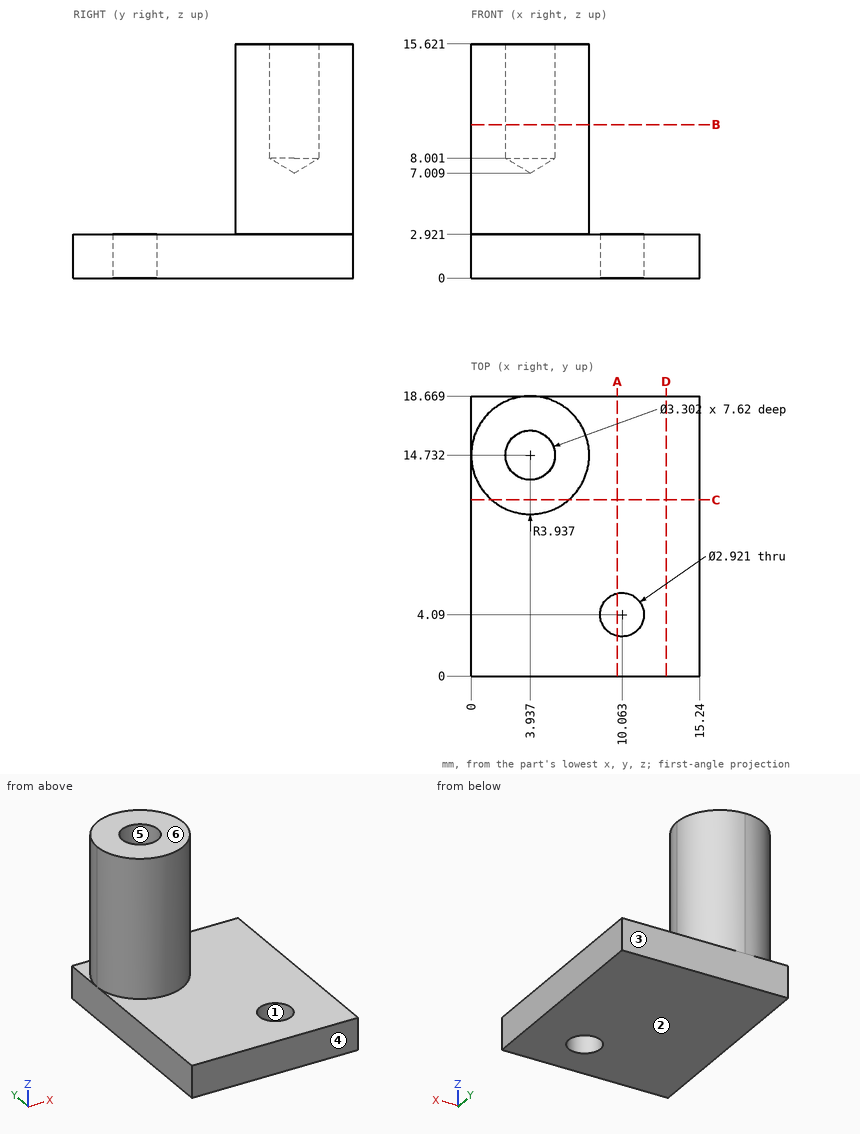
Job drawing, mm, ordinate dimensions from the low corner. One solid piece. A direction names the side the tool comes from. Round coordinates to 2 decimals unless told otherwise and drop trailing zeros. Loops run counter-clockwise (first coordinate to the right, second up) from the corner with the lowest first, then second, coordinate; pieces in that order, holes last. Notation, with made-up numbers: (87, -9) -> (119, -9) arc R25 cw to (119, 12) -> close; hole circle Ø6 at (-39, -25.5). An arc over 180 degrees is marked (long way). One line per item, written item: value. Start each with the question number.
Q1. Probe line 1 along Z through (x, y) = (12, 10.5); line 2 along X through (y, z) = (15.5, 7.75) (1 decimal); line 3 along X through (y, z) = (15, 8.75) (1 decimal). List the from-to ranges inside material, lowest first.
Q2. Two-plate mould, pull along Y, no slides. Class the marked faces 1, 2, 3 and 4: released by +Y, released by -Y, zero draft, split by the parting line, or undercut.
Q3. Cut at D-D on x = 13. List the corners of the cut face in (y, z).
Q4. Cut at B-B on z = 10.25. List the corners of the cut face in (x, y).
Q5. Cut at C-C on y = 11.75. List the corners of the cut face in (x, z).
Q6. 3-axis set-ups, long thin cutter, end or side, ignore diameter. For the marked faces 5 and 6: which of +Z, -Z, +X, -X, +Y, -Y reach the whole face in a straight line?
Q7. Cut at A-A on x = 9.75. List the corners of the cut face in (y, z).
Q8. Drop flat-ended pins along their axis: pin 1 Ø2 at (x, z) = (3, 6.5) entering from +Y; pin 2 Ø6 at (x, y) = (12.5, 12.5) entering from +Z; pin 3 Ø1.5 at (y, z) = (11, 11) entering from -X. Give the stop position or say it passes through.
Computed:
1. line 1: 0 to 2.92
1. line 2: 0.1 to 3, 4.9 to 7.8
1. line 3: 0 to 2.3, 5.6 to 7.9
2. face 1: undercut
2. face 2: zero draft
2. face 3: released by +Y
2. face 4: released by -Y
3. outline: (0, 0) -> (18.67, 0) -> (18.67, 2.92) -> (0, 2.92) -> close
4. outline: circle Ø7.87 at (3.94, 14.73); hole circle Ø3.3 at (3.94, 14.73)
5. outline: (0, 0) -> (15.24, 0) -> (15.24, 2.92) -> (6.51, 2.92) -> (6.51, 15.62) -> (1.37, 15.62) -> (1.37, 2.92) -> (0, 2.92) -> close
6. face 5: +Z
6. face 6: +Z, +X, -X, +Y, -Y
7. outline: (0, 0) -> (2.66, 0) -> (2.66, 2.92) -> (0, 2.92) -> close; (5.52, 0) -> (18.67, 0) -> (18.67, 2.92) -> (5.52, 2.92) -> close
8. pin 1: y = 18.67
8. pin 2: z = 2.92
8. pin 3: x = 1.37
